Autodesk Fusion 360 part; units mm, degrees
sketch "Skizze1" plane through (0, 0, 0) normal (0, 0, 1) x (1, 0, 0)
  circle A0 centre (0, 0) radius 15
  circle A1 centre (0, 0) radius 1.7
  circle A2 centre (0, 0) radius 7.55
  line L0 (0, 17.9163) -> (0, -17.3071) construction
  circle A3 centre (0, 0) radius 9.2 construction
  circle A4 centre (0, 9.2) radius 1.2
  circle A5 centre (0, -9.2) radius 1.2
  circle A6 centre (0, 0) radius 5
  circle A7 centre (0, 0) radius 14.1421 construction
  line L1 (9.2, -0.85) -> (7.502, -0.85)
  line L2 (9.2, 0.85) -> (7.502, 0.85)
  line L3 (19.7442, 0) -> (-23.5704, 0) construction
  line L4 (-4.9272, -0.85) -> (-9.2, -0.85)
  line L5 (-4.9272, 0.85) -> (-9.2, 0.85)
  line L6 (-9.2, -0.85) -> (-9.2, 0.85)
  line L7 (9.2, -0.85) -> (9.2, 0.85)
  circle A8 centre (0, 0) radius 8
  point P0 (0, 9.2)
  point P1 (0, -9.2)
  dimension "d1" = 30
  dimension "d2" = 3.4
  dimension "d3" = 15.1
  dimension "d19" = 18.4
  dimension "d20" = 2.4
  dimension "d21" = 2.4
  dimension "d25" = 10
  dimension "d43" = 28.2843
  dimension "d58" = 0.85
  dimension "d59" = 0.85
  dimension "d60" = 0.85
  dimension "d61" = 0.85
  dimension "d62" = 9.2
  dimension "d63" = 9.2
  dimension "d66" = 16
extrude "Extrusion1" add sketch "Skizze1" along normal blind 15 contours A1 | A6 makes body 1
extrude "Extrusion2" cut sketch "Skizze1" along normal blind 14 contours A1 bodies 1
extrude "Extrusion5" add sketch "Skizze1" along normal blind 12.7 contours A2 A6 L4 L5 | A2 A6 L4 L5 bodies 1
extrude "Extrusion9" add sketch "Skizze1" along normal blind 11.2 contours A2 L1 L2 A8 | A2 L4 L5 A8 | L1 L2 L7 A8 | L4 L5 L6 A8 bodies 1
extrude "Extrusion3" add sketch "Skizze1" along normal blind 9.3 separate body contours A0 | A2 L1 L2 A8 | A2 L4 L5 A8 | L1 L2 L7 A8 | L4 L5 L6 A8 makes body 2
extrude "Extrusion10" add sketch "Skizze1" along normal blind 8.8 contours A2 L2 L5 A8 | A2 L1 L4 A8 bodies 1 2
ref_plane "Arbeitsebene1" through (0, 0, 7.5) normal (0, 0, -1) x (-1, 0, 0)
sketch "Skizze2" plane through (0, 0, 7.5) normal (0, 0, -1) x (-1, 0, 0)
  line L0 (0, 19.4975) -> (0, -17.4097) construction
  line L1 (-20.2047, 0) -> (24.515, 0) construction
  circle A0 centre (0, 0) radius 9.2 construction
  line L2 (-1.3568, 11.55) -> (-2.7135, 9.2)
  line L3 (-2.7135, 9.2) -> (-1.3568, 6.85)
  line L4 (-1.3568, 6.85) -> (1.3568, 6.85)
  line L5 (1.3568, 6.85) -> (2.7135, 9.2)
  line L6 (2.7135, 9.2) -> (1.3568, 11.55)
  line L7 (1.3568, 11.55) -> (-1.3568, 11.55)
  line L8 (1.3568, -11.55) -> (2.7135, -9.2)
  line L9 (2.7135, -9.2) -> (1.3568, -6.85)
  line L10 (1.3568, -6.85) -> (-1.3568, -6.85)
  line L11 (-1.3568, -6.85) -> (-2.7135, -9.2)
  line L12 (-2.7135, -9.2) -> (-1.3568, -11.55)
  line L13 (-1.3568, -11.55) -> (1.3568, -11.55)
  point P0 (0, 9.2)
  point P1 (0, -9.2)
  point P2 (0, 9.2)
  point P3 (0, -9.2)
  dimension "d9" = 18.4
  dimension "d10" = 4.7
  dimension "d11" = 4.7
extrude "Extrusion4" cut sketch "Skizze2" against normal blind 2.1 bodies 1
chamfer "Fase2" distance 1 angle 45 1 edges at (-4.6616, -1.8081, 15) on bodies 1
Source: CAD feature listing. Evaluate the final solid. Frame: model axes, mm. A direction names the side the tool comes from. Round coordinates to 2 decimals unless told otherwise and drop trailing zeros. Loops run counter-clockwise (first coordinate to the right, second up) from the corner with the lowest first, then second, coordinate; pieces in that order, holes last. Notation, with made-up numbers: M 87,16.25 L 130,16.25 A15 cw 130,38.25 Z; hole C 67.25,-1 d9. An arc over 180 degrees is marked long. Answer as CSV lines item,"result".
Q1. Pull-direction query (X, two-part tool) for faces 3 (the face through (-2.045, -8.041, 8.535)), 4 (the face through (0, 0, 15)), 5 (the face through (-9.2, 0, 10)); classes: +X half, -X half, draft (parallel to the pull), parting line (faces both ways), or undercut.
Verdict:
face 3,"undercut"
face 4,"draft"
face 5,"-X half"
Q2. Cut plane C-C (y = 0). Return the cut outline in (x, z), plus the area to 3 significant figures.
Verdict:
outline,"M -15,0 L -1.7,0 L -1.7,14 L 1.7,14 L 1.7,0 L 15,0 L 15,9.3 L 9.2,9.3 L 9.2,11.2 L 7.55,11.2 L 7.55,12.7 L 5,12.7 L 5,14 L 4,15 L -4,15 L -5,14 L -5,12.7 L -7.55,12.7 L -7.55,11.2 L -9.2,11.2 L -9.2,9.3 L -15,9.3 Z"
area,"311 mm^2"
Q3. Contact query for flat-ended pins moving along their axis: pin 1 (1.4 mm diameter, centred on x = -8, y = 0.5, fed in from +Z); pin 2 (0.8 mm diameter, centred on y = 0.5, z = 10, fed in from +X); pin 3 (1.9 mm diameter, centred on x = -8, z = 9.5, fed in from +Y). Output: stop coordinate, or through.
Verdict:
pin 1,"stops at z = 12.7"
pin 2,"stops at x = 9.2"
pin 3,"stops at y = 13.23"
Q4. Cut plane A-A (x = 0). Count the separate pieces of the cut face and the enclosed holes in it, plus the area to 3 significant figures.
Verdict:
separate pieces,"3"
enclosed holes,"0"
area,"251 mm^2"
Q5. Cut plane B-B (z = 6.25). Return the cut outline in (x, y), plus the area to 3 significant figures.
Verdict:
outline,"C 0,0 d30; hole C 0,0 d3.4; hole C 0,-9.2 d2.4; hole C 0,9.2 d2.4"
area,"689 mm^2"
Q6. Line query: line 1 along Y through (x, z) = (0, 5.75); line 2 along Z through (x, y) = (-4.75, -2.5); line 3 along Z through (x, y) = (10.75, 9.25). Output: solid intervals per line, ascending.
Verdict:
line 1,"y = -15 to -10.4, -8 to -1.7, 1.7 to 8, 10.4 to 15"
line 2,"z = 0 to 12.7"
line 3,"z = 0 to 9.3"
Q7. Cut plane D-D (y = -6). Return the cut outline in (x, z).
Verdict:
outline,"M -13.75,0 L 13.75,0 L 13.75,9.3 L 5.29,9.3 L 5.29,8.8 L 4.58,8.8 L 4.58,12.7 L -4.58,12.7 L -4.58,8.8 L -5.29,8.8 L -5.29,9.3 L -13.75,9.3 Z"
Q8. Reachability of faces 1 (the face through (3, 0, 0)), 2 (the face through (6, -6, 9.3)) from +Z, -Z, +X, -X, +Y, -Y: full face, straight path, thin tool, end or side. Return the list, or none.
Verdict:
face 1,"-Z, +X, -X, +Y, -Y"
face 2,"+Z"
